For this review, use the dimensioned drawing (mm, ordinates from the lowest corner) and the shaded views. A direction names the side the tool comes from. Round coordinates to 2 decimals unless told otherwise and drop trailing zeros. Write each loop counter-clockwise with the first axis right and the second up, starting at its lowest first coordinate (ties: lowest second). Pieces come first, ordered by that corner, then holes.
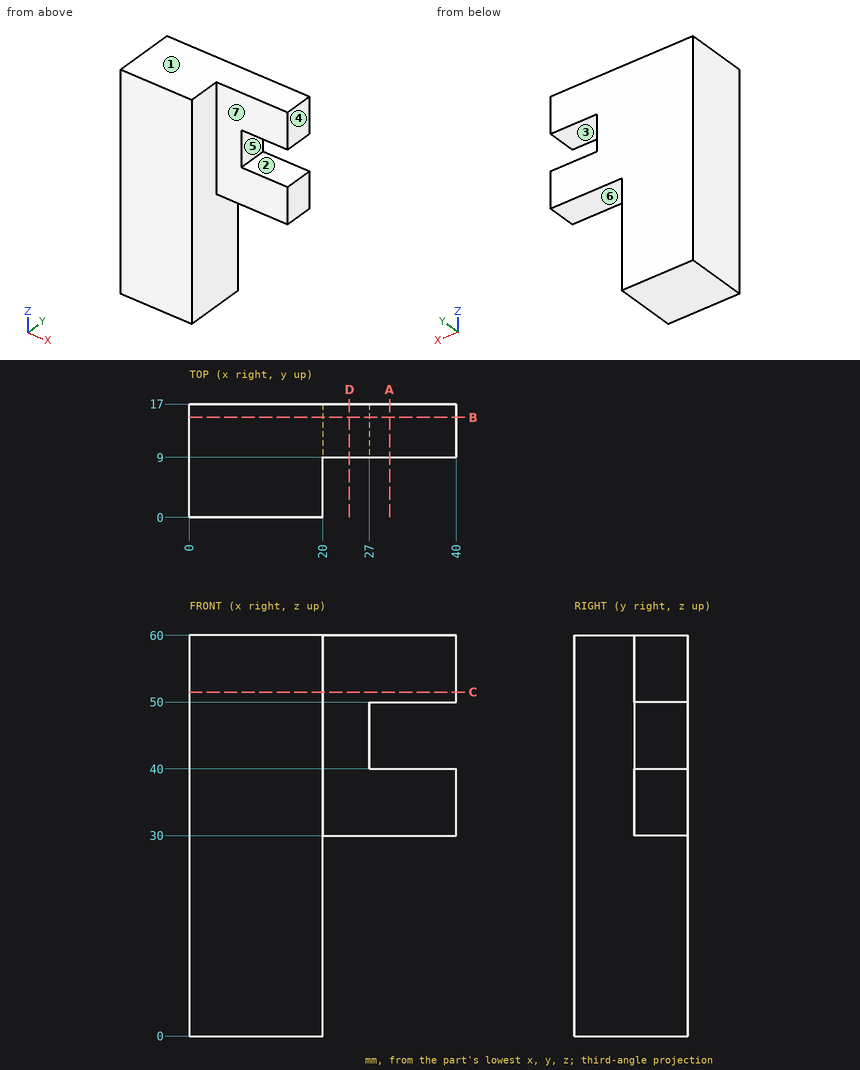
(1) We need section C-C, the plane z = 51.5. Give the boundary of the cut face in (x, y).
Geometry check:
outline: (0, 0) - (20, 0) - (20, 9) - (40, 9) - (40, 17) - (0, 17) - close
(2) For line 1 along Z through (x, y) = (28.5, 15); line 2 along Y through (x, z) = (21.5, 56); line 3 along X through (y, z) = (3, 48), list the stretches that pass through material, from the lowest coordinate up.
Geometry check:
line 1: z = 30 to 40, 50 to 60
line 2: y = 9 to 17
line 3: x = 0 to 20
(3) We need section A-A, the plane x = 30. Give the boundary of the cut face in (y, z).
Geometry check:
outline: (9, 30) - (17, 30) - (17, 40) - (9, 40) - close; (9, 50) - (17, 50) - (17, 60) - (9, 60) - close
(4) We need section D-D, the plane x = 24. Give the boundary of the cut face in (y, z), and give its area (3 significant figures).
Geometry check:
outline: (9, 30) - (17, 30) - (17, 60) - (9, 60) - close
area: 240 mm2
(5) For the marked faces 5, 6 and 7, list the 3-axis set-ups (+Z, -Z, +X, -X, +Y, -Y) from which the entire face can be reached by the end or side of a thin tool; tool diameter is ignored.
Geometry check:
face 5: +X, +Y, -Y
face 6: -Z, +X, +Y, -Y
face 7: +Z, -Z, +X, -Y
(6) Mouldability with a two-part tool opening along Z and no side actions: class the marked faces 1, 2, 3 and 4 as pulls with the +Z half, pulls with the -Z half, needs draft (parallel to the pull), parting line crosses it, or undercut.
Geometry check:
face 1: pulls with the +Z half
face 2: undercut
face 3: undercut
face 4: needs draft
(7) We need section B-B, the plane y = 15. Give the boundary of the cut face in (x, z).
Geometry check:
outline: (0, 0) - (20, 0) - (20, 30) - (40, 30) - (40, 40) - (27, 40) - (27, 50) - (40, 50) - (40, 60) - (0, 60) - close
(8) For pin 1 Ø3 at (x, y) = (15.5, 7.5) entering from -Z; pin 2 Ø3 at (x, y) = (32.5, 10.5) entering from -Z; pin 3 Ø6.5 at (y, z) = (13, 46) entering from +X, all flat-tipped, find the tip position at first contact; note any pin that passes through.
Geometry check:
pin 1: stops at z = 0
pin 2: stops at z = 30
pin 3: stops at x = 27
